Read the model definition and answer for the solid it produces. Units are mm, in the model's axes. Round coordinates to 2 decimals unless told otherwise and drop trailing zeros. Loops run counter-clockwise (first coordinate to the right, second up) from the corner with the lowest first, then second, coordinate; pieces in that order, holes last. Notation, with made-up numbers: (-24, 83) - (29, 83) arc R34 ccw to (29, 116) - close; hole circle Ø7 at (36.25, 73). An arc over 180 degrees is marked (long way). Use one line per item in the form item = value. Start each with the question number.
Solid Edge part; units mm, degrees
sketch "Sketch1" plane through (0, 0, 0) normal (0, 0, 1) x (1, 0, 0)
  line L0 (-140.5, -5.5) -> (-129.5, -5.5)
  line L1 (-129.5, -5.5) -> (-129.5, 5.5)
  line L2 (-129.5, 5.5) -> (-140.5, 5.5)
  line L3 (-140.5, 5.5) -> (-140.5, -5.5)
  line L4 (-5.5, -5.5) -> (5.5, -5.5)
  line L5 (5.5, -5.5) -> (5.5, 5.5)
  line L6 (5.5, 5.5) -> (-5.5, 5.5)
  line L7 (-5.5, 5.5) -> (-5.5, -5.5)
extrude "ExtrudedProtrusion_1" add sketch "Sketch1" along normal blind 35
sketch "Sketch2" plane through (-129.5, 0, 17.5) normal (1, 0, 0) x (0, 1, 0)
  line L0 (-5.5, 17.5) -> (5.5, 8.2699)
  line L1 (5.5, 8.2699) -> (8.7139, 12.1001)
  line L2 (-2.2861, 21.3302) -> (8.7139, 12.1001)
  line L3 (-5.5, 17.5) -> (-2.2861, 21.3302)
extrude "Protrusion1" add sketch "Sketch2" along normal up to vertex (124 mm away)
sketch "Sketch3" plane through (-135, 0, 35) normal (0, 0, 1) x (1, 0, 0)
  line L0 (5.5, -5.5) -> (-5.5, -5.5)
  line L1 (-5.5, -5.5) -> (-5.5, 5.5)
  line L2 (-5.5, 5.5) -> (5.5, 5.5)
  line L3 (5.5, 5.5) -> (5.5, -5.5)
  line L4 (140.5, -5.5) -> (129.5, -5.5)
  line L5 (129.5, -5.5) -> (129.5, 5.5)
  line L6 (129.5, 5.5) -> (140.5, 5.5)
  line L7 (140.5, 5.5) -> (140.5, -5.5)
extrude "Protrusion2" add sketch "Sketch3" along normal up to vertex (3.8302 mm away)
sketch "Sketch4" plane through (-129.5, 0, 17.5) normal (1, 0, 0) x (0, 1, 0)
  line L0 (8.7139, 12.1001) -> (-2.2861, 21.3302)
  line L1 (-5.5, 17.5) -> (-2.2861, 21.3302)
  line L2 (5.5, 8.2699) -> (-5.5, 17.5)
extrude "ExtrudedCutout_1" cut sketch "Sketch4" against normal blind 22.2856 and the other way blind 177.6733 material side at (-129.5, 3.246, 34.2535)
sketch "Sketch5" plane through (-129.5, -3.893, 36.9151) normal (1, 0, 0) x (0, 1, 0)
  line L0 (-1.607, 1.9151) -> (-1.607, -1.9151)
  line L1 (-1.607, -1.9151) -> (1.607, 1.9151)
  line L2 (1.607, 1.9151) -> (-1.607, 1.9151)
extrude "Protrusion3" add sketch "Sketch5" along normal up to vertex (124 mm away)
sketch "Sketch6" plane through (-5.5, 7.107, 29.0334) normal (1, 0, 0) x (0, 0.7660444, -0.6427876)
  line L0 (-3.3288, 1.4671) -> (0.8667, -3.5329)
  line L1 (0.8667, -3.5329) -> (0.8667, 1.4671)
  line L2 (0.8667, 1.4671) -> (-3.3288, 1.4671)
extrude "ExtrudedCutout_2" cut sketch "Sketch6" against normal blind 148.825
chamfer "Chamfer_1" distance 2 angle 45 2 edges at (5.5, 5.5, 29.0334) (-140.5, 5.5, 29.0334)
sketch "Sketch7" plane through (-5.5, -3.893, 36.9151) normal (1, 0, 0) x (0, 1, 0)
  line L0 (-1.607, 1.9151) -> (-1.607, -1.9151)
  line L1 (-1.607, -1.9151) -> (1.607, 1.9151)
  line L2 (1.607, 1.9151) -> (-1.607, 1.9151)
extrude "ExtrudedCutout_3" cut sketch "Sketch7" against normal blind 147.0502
1) A cutting plane is placed at B-B on x = -126. Write down the section's boundary in (y, z), plus the area to 3 significant figures.
2) Straight lines are drawn through the part: line 1 (Y direction, x = -92, z = 37); line 2 (Z direction, x = -96, y = 1.75); line 3 (Y direction, x = -114, z = 34.5). For each, find the intervals that lie inside material, in ascending order. Write a range as from..to.
3) Determine the mould class of faces 1 (the flat face through (-66.48, -0.08, 30.45)), 2 (the flat face through (5.5, 0, 33)), 3 (the flat face through (-66.48, 1.55, 35.61)) for opening direction Y: +Y half, -Y half, draft (parallel to the pull), parting line (faces both ways), or undercut.
4) A cutting plane is placed at A-A on y = 1.5. Write down the section's boundary in (x, z), plus the area to 3 significant figures.
5) Flat-ended cylindrical pins translate along their axes: pin 1 (6 mm diameter, centred on x = -94.5, z = 32.5, fed in from -Y); pin 2 (3 mm diameter, centred on y = -3.5, z = 31.5, fed in from +X); pin 3 (6 mm diameter, centred on x = -29.5, y = -2, fed in from -Z). Find the tip coordinate at first contact, or state that the pin passes through.
Checks:
q1.outline = (-5.5, 35) - (5.5, 25.77) - (5.5, 32.3) - (-2.29, 38.83) - close
q1.area = 61.3 mm²
q2.line_1 = -3.82..-0.1
q2.line_2 = 28.92..35.44
q2.line_3 = -4.9..2.87
q3.face_1 = -Y half
q3.face_2 = draft
q3.face_3 = +Y half
q4.outline = (-140.5, 29.13) - (5.5, 29.13) - (5.5, 35.65) - (-140.5, 35.65) - close
q4.area = 953 mm²
q5.pin_1 = -5.5
q5.pin_2 = 5.5
q5.pin_3 = 29.55
